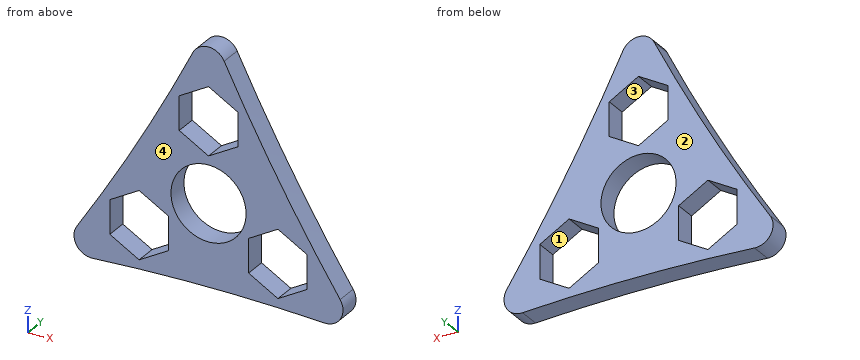
```python
from build123d import *

# Parameters (mm, degrees)
F0_R     = 10.9
F1_DEPTH = 6.35
F2_R     = 5.08


with BuildPart() as f1:
    # F0 (on Front) → F1 (new body)
    with BuildSketch(Plane.XZ):
        with BuildLine():
            ThreePointArc((0, 50.8), (-20.4902984868, 11.8300793471), (-43.9940905122, -25.4))
            ThreePointArc((-43.9940905122, -25.4), (0, -23.6601586942), (43.9940905122, -25.4))
            ThreePointArc((43.9940905122, -25.4), (20.4902984868, 11.8300793471), (0, 50.8))
        make_face()
        Polygon((-11.6393814269, -16.5349545762), (-20.1393814269, -21.4424318643), (-28.6393814269, -16.5349545762), (-28.6393814269, -6.72), (-20.1393814269, -1.8125227119), (-11.6393814269, -6.72), align=None, mode=Mode.SUBTRACT)
        Circle(F0_R, mode=Mode.SUBTRACT)
        Polygon((20.1393814269, -1.8125227119), (28.6393814269, -6.72), (28.6393814269, -16.5349545762), (20.1393814269, -21.4424318643), (11.6393814269, -16.5349545762), (11.6393814269, -6.72), align=None, mode=Mode.SUBTRACT)
        Polygon((0, 13.44), (-8.5, 18.3474772881), (-8.5, 28.1624318643), (0, 33.0699091524), (8.5, 28.1624318643), (8.5, 18.3474772881), align=None, mode=Mode.SUBTRACT)
    extrude(amount=F1_DEPTH)

    # F2
    f2_edges = [f1.edges().sort_by_distance(p)[0] for p in [
        (-43.994091, -3.175, -25.4),
        (43.994091, -3.175, -25.4),
        (0, -3.175, 50.8),
    ]]
    fillet(f2_edges, radius=F2_R)


solid = f1.part
```
For this review, take the finished solid that the model builds, in its own axes (mm). Face numbers are marked on the shaded views. A direction names the side the tool comes from. Round coordinates to 2 decimals unless told otherwise and drop trailing zeros. Loops run counter-clockwise (first coordinate to the right, second up) from the corner with the lowest first, then second, coordinate; pieces in that order, holes last.
(1) Mouldability with a two-part tool opening along X and no side actions: class the marked faces 3 and 4 as released by +X, released by -X, zero draft, split by the parting line, or undercut.
Returned:
face 3: undercut
face 4: zero draft
(2) We need section A-A (z = 5). Give the boundary of the cut face in (x, y), plus the area to 3 significant figures.
Returned:
outline: (-24.5, -6.35) - (-9.69, -6.35) - (-9.69, 0) - (-24.5, 0) - close; (9.69, -6.35) - (24.5, -6.35) - (24.5, 0) - (9.69, 0) - close
area: 188 mm2
(3) Tool access review of the marked faces 1 and 2: name each direction out of +Z, -Z, +X, -X, +Y, -Y from which nothing blocks a thin tool from reaching the whole face with its end or side.
Returned:
face 1: +Y, -Y
face 2: +Z, -Z, +X, -X, +Y
(4) Clearance check with flat-ended pins moving along their axes: P1, Ø1.9, axis at y = -4.5, z = 23.5, coming from the +X side; P2, Ø4, axis at x = 9.5, z = -16.5, coming from the +Y side; P3, Ø1.9, axis at y = -2.5, z = 21.5, coming from the -X side; P4, Ø3, axis at y = -1.5, z = -12, coming from the +X side. State where each tip first meets the part, or that it passes through.
Returned:
P1: stops at x = 14.46
P2: stops at y = 0
P3: stops at x = -15.56
P4: stops at x = 36.03
(5) We need section B-B (x = 25). Give the boundary of the cut face in (y, z), plus the area to 3 significant figures.
Returned:
outline: (-6.35, -24.22) - (0, -24.22) - (0, -18.64) - (-6.35, -18.64) - close; (-6.35, -4.62) - (0, -4.62) - (0, 4.16) - (-6.35, 4.16) - close
area: 91.2 mm2
(6) We need section C-C (y = -2.5). State how many separate pieces and enclosed holes the cut face has, plus the area to 3 significant figures.
Returned:
separate pieces: 1
enclosed holes: 4
area: 1,850 mm2
(7) Wall thickness on line 1 along Z through (x, y) = (0, -4.75); line 2 along X through (y, z) = (-1, -4); line 3 along X through (y, z) = (-4.5, -12.5): over which ranges is each line inside the solid? List them lowest first.
Returned:
line 1: z = -23.66 to -10.9, 10.9 to 13.44, 33.07 to 44.29
line 2: x = -29.98 to -23.93, -16.35 to -10.14, 10.14 to 16.35, 23.93 to 29.98
line 3: x = -35.38 to -28.64, -11.64 to 11.64, 28.64 to 35.38
